Check sheet for the modelled part. Datum: model origin and axes. Units: mm. Face numbers are marked on the shaded views. A direction names the side the tool comes from. Coordinates: 2 decimals unless noted, no trailing zeros. Loops run counter-clockwise (first coordinate to the right, second up) from the corner with the lowest first, then second, coordinate; pieces in that order, holes last. Notation, with made-up numbers: M -22.5,55.5 L -9.5,55.5 A19 cw -9.5,66.5 Z; hole C 61,54.5 d7. An arc over 180 degrees is marked long. Use CSV: the item, a comma, the result in double quotes. Start each with the question number.
(1) Section check A-A on x = 9.5. Record the cut outline in (y, z), and give its area (3 significant figures).
(2) Draft check along Y on the marked faces 3, 4 and 5. Enter one of: pulls with the +Y half, pulls with the -Y half, needs draft (parallel to the pull), parting line crosses it, or undercut.
(3) Set-up check for the marked faces 1 and 2: record each of +Z, -Z, +X, -X, +Y, -Y from which the full face is reachable in a straight line by a thin tool's end or side.
(4) Section check C-C on x = -8.5. Record the cut outline in (y, z).
(5) Scan lines: line 1 (X direction, y = 0, z = 79); line 2 (Y direction, x = 18.8, z = -0.45); line 3 (Y direction, x = -20, z = 29). Record each from-to range of solid material in increasing order.
(6) Section check B-B on z = 50. Record the cut outline in (x, y), and give its area (3 significant figures).
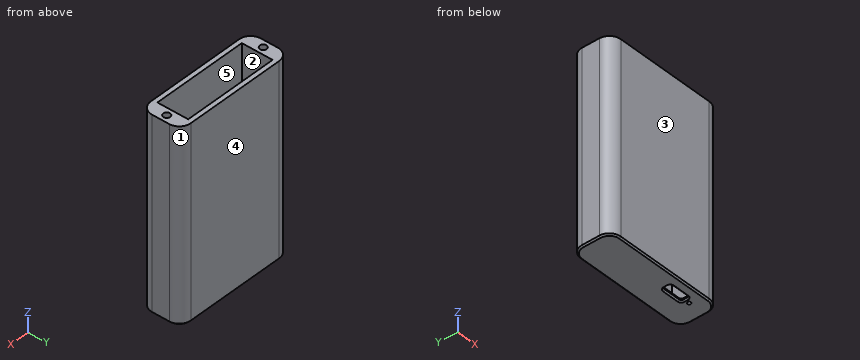
Autodesk Inventor part; units mm, degrees
ref_plane "YZ Plane" through (0, 0, 0) normal (1, 0, 0) x (0, 1, 0)
ref_plane "XZ Plane" through (0, 0, 0) normal (0, 1, 0) x (-1, 0, 0)
ref_plane "XY Plane" through (0, 0, 0) normal (0, 0, 1) x (1, 0, 0)
sketch "Sketch1" plane through (0, 0, 0) normal (0, 0, 1) x (1, 0, 0)
  point P0 (0, 0)
sketch "Sketch2" plane through (0, 0, 0) normal (0, 0, 1) x (1, 0, 0)
  line L0 (-21, 6.75) -> (21, 6.75)
  line L1 (21, 6.75) -> (21, -6.75)
  line L2 (21, -6.75) -> (-21, -6.75)
  line L3 (-21, -6.75) -> (-21, 6.75)
  line L4 (-27, 8.75) -> (27, 8.75)
  line L5 (27, 8.75) -> (27, -8.75)
  line L6 (27, -8.75) -> (-27, -8.75)
  line L7 (-27, -8.75) -> (-27, 8.75)
  point P0 (0, 0)
  dimension "d0" = 42
  dimension "d1" = 13.5
  dimension "d2" = 2
  dimension "d3" = 2
  dimension "d4" = 6
  dimension "d5" = 6
  dimension "d6" = 6.75
  dimension "d7" = 21
extrude "Extrusion1" add sketch "Sketch2" along normal blind 82
sketch "Sketch3" plane through (0, 0, 0) normal (0, 0, -1) x (-1, 0, 0)
  line L0 (-27, -8.75) -> (-27, 8.75)
  line L1 (27, 8.75) -> (27, -8.75)
  line L2 (-27, 8.75) -> (27, 8.75)
  line L3 (27, 8.75) -> (27, -8.75)
  line L4 (27, -8.75) -> (-27, -8.75)
  line L5 (-27, -8.75) -> (-27, 8.75)
  point P0 (0, 0)
extrude "Extrusion2" add sketch "Sketch3" along normal blind 1.2
fillet "Fillet1" radius 5 4 edges at (-27, 8.75, 40.4) (-27, -8.75, 40.4) (27, 8.75, 40.4) (27, -8.75, 40.4)
sketch "Sketch4" plane through (0, 0, 82) normal (0, 0, 1) x (1, 0, 0)
  line L0 (-21, -6.75) -> (-21, 6.75)
  line L1 (21, 6.75) -> (21, -6.75)
  line L2 (21, -6.75) -> (-21, -6.75)
  point P0 (0, 0)
  point P1 (-24, 0)
  point P2 (24, 0)
  dimension "d13" = 3
  dimension "d14" = 3
  dimension "d15" = 6.75
  dimension "d16" = 6.75
hole "Hole1" at (-24, 0, 82) at (24, 0, 82) direction (0, 0, -1) diameter 3 depth 8.8 tip angle 118
sketch "Sketch5" plane through (0, 0, 0) normal (0, 0, 1) x (1, 0, 0)
  line L0 (7.5, -1.05) -> (16.7, -1.05)
  line L1 (16.7, -1.05) -> (16.7, -4.55)
  line L2 (16.7, -4.55) -> (7.5, -4.55)
  line L3 (7.5, -4.55) -> (7.5, -1.05)
  line L4 (21, -6.75) -> (-21, -6.75)
  line L5 (21, 6.75) -> (21, -6.75)
  point P0 (0, 0)
  dimension "d24" = 2.2
  dimension "d25" = 3.5
  dimension "d26" = 9.2
  dimension "d27" = 4.3
extrude "Extrusion3" cut sketch "Sketch5" against normal blind 1.2
fillet "Fillet2" radius 1 4 edges at (16.7, -1.05, -0.6) (16.7, -4.55, -0.6) (7.5, -4.55, -0.6) (7.5, -1.05, -0.6)
sketch "Sketch6" plane through (0, 0, 0) normal (0, 0, 1) x (1, 0, 0)
  circle A0 centre (18.8, -2.8) radius 0.75
  line L0 (21, 6.75) -> (21, -6.75)
  line L1 (15.7, -4.55) -> (8.5, -4.55)
  line L2 (8.5, -1.05) -> (15.7, -1.05)
  point P0 (0, 0)
  dimension "d31" = 1.5
  dimension "d32" = 2.2
  dimension "d33" = 1.75
  dimension "d34" = 1.75
extrude "Extrusion4" cut sketch "Sketch6" against normal blind 1.2
chamfer "Chamfer1" distance 0.6 angle 45 8 edges at (12.1, -1.05, -1.2) (7.7929, -1.3429, -1.2) (7.5, -2.8, -1.2) (7.7929, -4.2571, -1.2) (12.1, -4.55, -1.2) (16.4071, -4.2571, -1.2) (16.7, -2.8, -1.2) (16.4071, -1.3429, -1.2)
chamfer "Chamfer2" distance 0.6 angle 45 8 edges at (0, 8.75, -1.2) (25.5355, 7.2855, -1.2) (27, 0, -1.2) (25.5355, -7.2855, -1.2) (0, -8.75, -1.2) (-25.5355, -7.2855, -1.2) (-27, 0, -1.2) (-25.5355, 7.2855, -1.2)
properties part number "base"
Outcome:
1,outline,"M -8.75,-0.6 L -8.15,-1.2 L -5.15,-1.2 L -4.55,-0.6 L -4.55,0 L -6.75,0 L -6.75,82 L -8.75,82 Z; M -1.05,-0.6 L -0.45,-1.2 L 8.15,-1.2 L 8.75,-0.6 L 8.75,82 L 6.75,82 L 6.75,0 L -1.05,0 Z"
1,area,"344 mm²"
2,face 3,"pulls with the -Y half"
2,face 4,"pulls with the +Y half"
2,face 5,"undercut"
3,face 1,"+Z, -Z, +X, +Y"
3,face 2,"+Z"
4,outline,"M -8.75,-0.6 L -8.15,-1.2 L 8.15,-1.2 L 8.75,-0.6 L 8.75,82 L 6.75,82 L 6.75,0 L -6.75,0 L -6.75,82 L -8.75,82 Z"
5,line 1,"x = -27 to -25.5, -22.5 to -21, 21 to 22.5, 25.5 to 27"
5,line 2,"y = -8.75 to -3.55, -2.05 to 8.75"
5,line 3,"y = -8.75 to -6.75, 6.75 to 8.75"
6,outline,"M -27,-3.75 A5 ccw -22,-8.75 L 22,-8.75 A5 ccw 27,-3.75 L 27,3.75 A5 ccw 22,8.75 L -22,8.75 A5 ccw -27,3.75 Z; hole M -21,-6.75 L 21,-6.75 L 21,6.75 L -21,6.75 Z"
6,area,"357 mm²"
